from build123d import *

# Parameters (mm, degrees)
F0_W      = 160
F0_H      = 14
F1_DEPTH  = 4.826
F2_W      = 4.826
F2_H      = 3
F3_DEPTH  = 4.826
F4_DEPTH  = 25
F5_R      = 0.5
F6_DEPTH  = 4.827
F8_DEPTH  = 4.827
F10_DEPTH = 4.827


with BuildPart() as f1:
    # F0 (on Top) → F1 (new body)
    with BuildSketch(Plane.XY):
        Rectangle(F0_W, F0_H)
    extrude(amount=F1_DEPTH)

    # F2 (on face) → F3 (join, through all)
    with BuildSketch(Plane.XY.offset(4.826)):
        with Locations((82.413, 5.5)):
            Rectangle(F2_W, F2_H)
        with Locations((82.413, -5.5)):
            Rectangle(F2_W, F2_H)
    extrude(amount=-F3_DEPTH)

    # F2 (on face) → F4 (cut)
    with BuildSketch(Plane.XY.offset(4.826)):
        Polygon((80, -1.55), (80, 1.55), (77.2, 1.55), (77.2, 2.9), (74.5, 2.9), (74.5, 1.55), (71.5, 1.55), (71.5, -1.55), (74.5, -1.55), (74.5, -2.9), (77.2, -2.9), (77.2, -1.55), align=None)
    extrude(amount=-F4_DEPTH, mode=Mode.SUBTRACT)

    # F5 (on face) → F6 (cut, through all)
    with BuildSketch(Plane.XY.offset(4.826)):
        with Locations((79.823223, 4.176777)):
            Circle(F5_R)
        with Locations((79.823223, -4.176777)):
            Circle(F5_R)
    extrude(amount=-F6_DEPTH, mode=Mode.SUBTRACT)

    # F7 (on face) → F8 (cut, through all)
    with BuildSketch(Plane.XY.offset(4.826)):
        with BuildLine():
            Line((-57.5, 3.5), (-72.5, 3.5))
            ThreePointArc((-72.5, 3.5), (-76, 0), (-72.5, -3.5))
            Line((-72.5, -3.5), (-57.5, -3.5))
            ThreePointArc((-57.5, -3.5), (-54, 0), (-57.5, 3.5))
        make_face()
    extrude(amount=-F8_DEPTH, mode=Mode.SUBTRACT)

    # F9 (on face) → F10 (cut, through all)
    with BuildSketch(Plane.XY.offset(4.826)):
        with BuildLine():
            ThreePointArc((-72.5, -7), (-79.5, 0), (-72.5, 7))
            Line((-72.5, 7), (-80, 7))
            Line((-80, 7), (-80, -7))
            Line((-80, -7), (-72.5, -7))
        make_face()
    extrude(amount=-F10_DEPTH, mode=Mode.SUBTRACT)


solid = f1.part
Model file for the job. Use its own axes, mm. A direction names the side the tool comes from. Coordinates: 2 decimals unless noted, no trailing zeros. Loops run counter-clockwise (first coordinate to the right, second up) from the corner with the lowest first, then second, coordinate; pieces in that order, holes last. Notation, with made-up numbers: (10.5, 73.25) -> (61.5, 73.25) arc R27 ccw to (61.5, 104.25) -> close; hole circle Ø7 at (-22.75, 13). An arc over 180 degrees is marked (long way). Use one line per item in the form item = value. Start each with the question number.
(1) Pull direction X, two halves, no side cores. Call faces 1 (the flat face through (76, -2.9, 2)), 2 (the flat face through (84.826, -6, 2)), 3 (the flat face through (79, -1.55, 2)): pulls with the +X half, pulls with the -X half, needs draft (parallel to the pull), parting line crosses it, or undercut.
(2) Cut at A-A on x = -64.5. Give the cut face in (y, z), and give its area (3 significant figures).
(3) Probe probe 1 along Y at (x, z) = (72, 0.75); probe 2 along X at (y, z) = (0, 2.7); probe 3 along Y at (x, z) = (77, 0.95). List the from-to ranges inside material, lowest first. Write a range as from..to.
(4) Cut at B-B on y = 0. Give the cut face in (x, z).
(5) Tool access for faces 4 (the flat face through (5, -7, 2)), 5 (the flat face through (83, 4, 2)), 6 (the cylindrical face through (-76, 0, 2)): list every direction of +Z, -Z, +X, -X, +Y, -Y with a clear straight run to the whole face (end or side of a thin tool).
(6) Flat gauge pins, fed straight in: pin 1 (0.7 mm diameter, centred on y = -2.5, z = 2.5, fed in from -X); pin 2 (0.7 mm diameter, centred on y = 2.5, z = 2.5, fed in from +X). Where does each tip first touch, or does it go through?
(7) Cut at C-C on z = 3.9. Give the cut face in (x, y).
Values:
q1.face_1 = undercut
q1.face_2 = pulls with the +X half
q1.face_3 = needs draft
q2.outline = (-7, 0) -> (-3.5, 0) -> (-3.5, 4.83) -> (-7, 4.83) -> close; (3.5, 0) -> (7, 0) -> (7, 4.83) -> (3.5, 4.83) -> close
q2.area = 33.8 mm2
q3.probe_1 = -7..-1.55, 1.55..7
q3.probe_2 = -79.5..-76, -54..71.5
q3.probe_3 = -7..-2.9, 2.9..7
q4.outline = (-79.5, 0) -> (-76, 0) -> (-76, 4.83) -> (-79.5, 4.83) -> close; (-54, 0) -> (71.5, 0) -> (71.5, 4.83) -> (-54, 4.83) -> close
q5.face_4 = +Z, -Z, +X, -X, -Y
q5.face_5 = +Z, -Z, +X
q5.face_6 = +Z, -Z
q6.pin_1 = -79.16
q6.pin_2 = 80
q7.outline = (-72.5, -7) -> (84.83, -7) -> (84.83, -4) -> (80.29, -4) arc R0.5 cw (long way) to (80, -3.71) -> (80, -1.55) -> (77.2, -1.55) -> (77.2, -2.9) -> (74.5, -2.9) -> (74.5, -1.55) -> (71.5, -1.55) -> (71.5, 1.55) -> (74.5, 1.55) -> (74.5, 2.9) -> (77.2, 2.9) -> (77.2, 1.55) -> (80, 1.55) -> (80, 3.71) arc R0.5 cw (long way) to (80.29, 4) -> (84.83, 4) -> (84.83, 7) -> (-72.5, 7) arc R7 ccw to start; hole (-72.5, -3.5) -> (-57.5, -3.5) arc R3.5 ccw to (-57.5, 3.5) -> (-72.5, 3.5) arc R3.5 ccw to start
